Can you work these out from the drawing? Everything is in mm from the part's minimum corner. Round coordinates to 2 decimals unless told otherwise and drop trailing zeros. Order: outer loops, then holes, each group sorted by start corner. A loop starts at its lowest first (then second) coordinate and runs counter-clockwise, first axis right, second up. Notation, with made-up numbers: (61.5, 41.5) - (105.5, 41.5) arc R24 cw to (105.5, 73.5) - close; hole circle Ø10 at (36, 65.5). An arc over 180 degrees is marked (long way). Answer as a JSON object with one key per item and string values.
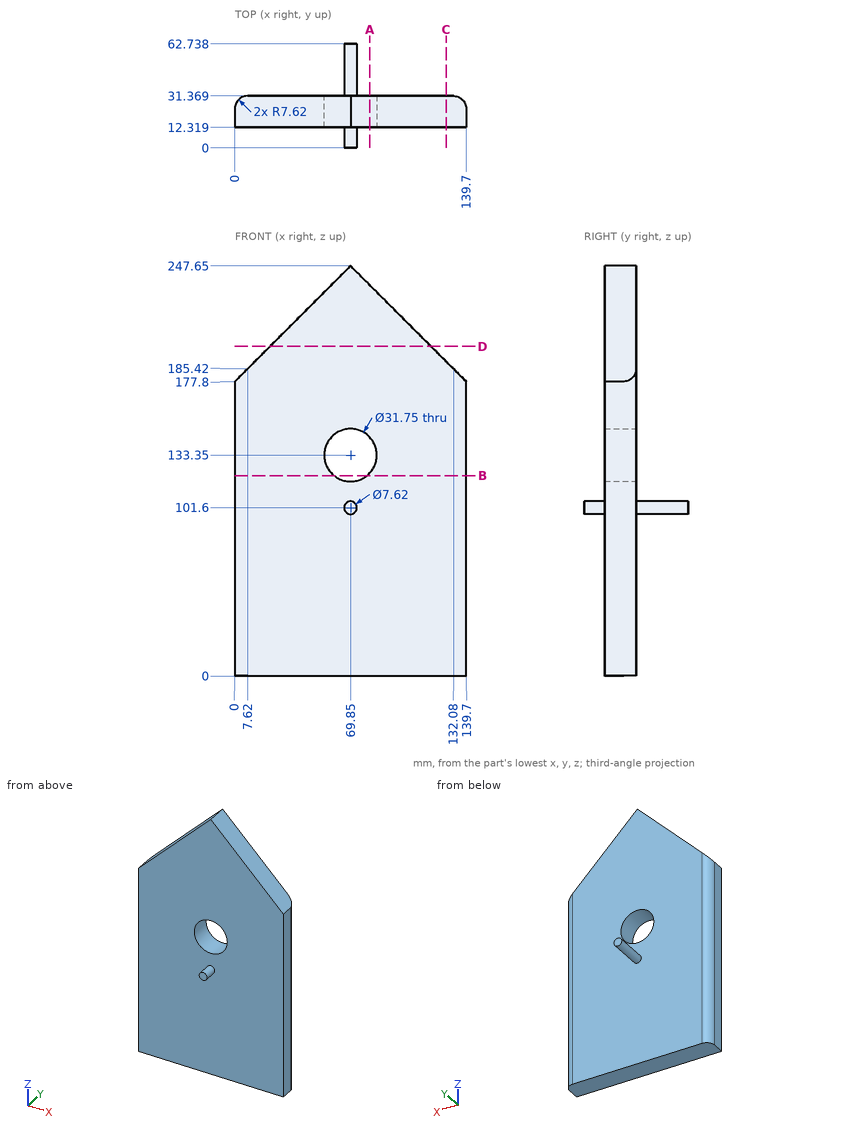
1. Imagine slicing it at C-C (x = 127.5). List the corners of the cut face in (y, z) for me.
Responses:
{"outline": "(12.32, 0) - (31.37, 0) - (31.37, 190) - (12.32, 190) - close"}
2. Imagine slicing it at A-A (x = 81.5). List the corners of the cut face in (y, z) for me, plus the area to 3 significant figures.
Responses:
{"outline": "(12.32, 0) - (31.37, 0) - (31.37, 122.57) - (12.32, 122.57) - close; (12.32, 144.13) - (31.37, 144.13) - (31.37, 236) - (12.32, 236) - close", "area": "4,080 mm2"}
3. Imagine slicing it at B-B (z = 121). List the corners of the cut face in (x, y) for me.
Responses:
{"outline": "(0, 12.32) - (59.88, 12.32) - (59.88, 31.37) - (7.62, 31.37) arc R7.62 ccw to (0, 23.75) - close; (79.82, 12.32) - (139.7, 12.32) - (139.7, 23.75) arc R7.62 ccw to (132.08, 31.37) - (79.82, 31.37) - close"}
4. Imagine slicing it at D-D (z = 199). List the corners of the cut face in (x, y) for me.
Responses:
{"outline": "(21.2, 12.32) - (118.5, 12.32) - (118.5, 31.37) - (21.2, 31.37) - close"}
5. If I drill on L1, parallel to Y at x = 100, z = 210; L2, parallel to Z at x = 70.5, y = 41.5; L3, parallel to X at y = 29.5, z = 29, over which ranges is the centre line in solid material (lowest first)? Write a range as [from, to].
Responses:
{"L1": "[12.32, 31.37]", "L2": "[97.85, 105.35]", "L3": "[2.62, 137.08]"}
6. For P1, Ø10, axis at x = 37.5, z = 143.5, coming from the +Y side; P2, Ø4, axis at x = 79.5, y = 16.5, coming from the +Z side; P3, Ø1.5, axis at x = 48.5, y = 14, coming from the +Z side, each with a flat end and sliding along its axis, tell me the tip position at first contact or that it passes through.
Responses:
{"P1": "y = 31.37", "P2": "z = 240", "P3": "z = 227.05"}
